Part model, mm, in its own coordinate system. A direction names the side the tool comes from. Give positions to 0.01 mm unless a question says otherwise; leave off trailing zeros. Write each loop counter-clockwise with the first axis right and the second up, starting at its lowest first coordinate (ties: lowest second). Pieces come first, ordered by that corner, then holes.
from build123d import *

# Parameters (mm, degrees)
ESQUISSE2_R                  = 20
BOSS_EXTRU_1_DEPTH           = 5
BOSS_EXTRU_2_DEPTH           = 5
R_P_TITION_CIRCULAIRE1_COUNT = 24
D_GAGEMENT_M22_D             = 5.1
BOSS_EXTRU_3_DEPTH           = 7.5
ENL_V_MAT_EXTRU_2_DEPTH      = 83.82071633
ENL_V_MAT_EXTRU_2_DEPTH_BACK = 83.82071633
ESQUISSE13_W                 = 57.206213055
ESQUISSE13_H                 = 37.798612504
ESQUISSE14_W                 = 4.5
ESQUISSE14_H                 = 4.5
BOSS_EXTRU_5_DEPTH           = 5
ESQUISSE17_W                 = 20
ESQUISSE17_H                 = 15
BOSS_EXTRU_7_DEPTH           = 2
CONG_1_R                     = 2
CONG_2_R                     = 2


with BuildPart() as part:
    # Esquisse2 → Boss.-Extru.1 (new body)
    with BuildSketch(Plane(origin=(0, 0, 0), x_dir=(1, 0, 0), z_dir=(0, 1, 0))):
        with Locations(Location((0, 0, 0), (0, 0, 270))):
            Circle(ESQUISSE2_R)
    extrude(amount=BOSS_EXTRU_1_DEPTH)

    # Esquisse3 → Boss.-Extru.2 (add)
    with BuildSketch(Plane(origin=(0, 5, 0), x_dir=(1, 0, 0), z_dir=(0, 1, 0))):
        Polygon((-1.625, 19.933875062), (-1.25, 21.933875062), (1.25, 21.933875062), (1.625, 19.933875062), align=None)
    boss_extru_2 = extrude(amount=-BOSS_EXTRU_2_DEPTH)

    # Répétition circulaire1: Boss.-Extru.2 ×24 about axis
    r_p_tition_circulaire1_axis = Axis((0, 0, 0), (0, 1, 0))
    for i in range(1, R_P_TITION_CIRCULAIRE1_COUNT):
        add(boss_extru_2.rotate(r_p_tition_circulaire1_axis, i * 360 / R_P_TITION_CIRCULAIRE1_COUNT))

    # Dégagement M22 (through all)
    with Locations(Plane(origin=(0, 5, 0), x_dir=(1, 0, 0), z_dir=(0, 1, 0))):
        with Locations((0, 0)):
            Hole(D_GAGEMENT_M22_D / 2)

    # Esquisse11 → Boss.-Extru.3 (add)
    with BuildSketch(Plane(origin=(0, 5, 0), x_dir=(1, 0, 0), z_dir=(0, 1, 0))):
        Polygon((-5.801101772, -14.332121903), (1.625908743, -15.37592016), (-0.461687771, -30.229941191), (3.284378163, -39.501779737), (-2.282545875, -79.112502486), (-6.738752185, -78.486223532), (-1.894992792, -44.021084607), (-7.888698287, -29.186142934), align=None)
    extrude(amount=-BOSS_EXTRU_3_DEPTH)

    # Esquisse13 → Enlèv. mat.-Extru.2 (cut, two sides: drawn at the far end of the back side and taken through both)
    with BuildSketch(Plane(origin=(3.713505258, 0, 0.521899129), x_dir=(0.13917310096006574, 0, -0.9902680687415703), z_dir=(0.9902680687415703, 0, 0.13917310096006574)).offset(-ENL_V_MAT_EXTRU_2_DEPTH_BACK)):
        with Locations((6.964953995, 7.661661133)):
            Rectangle(ESQUISSE13_W, ESQUISSE13_H)
    extrude(amount=ENL_V_MAT_EXTRU_2_DEPTH + ENL_V_MAT_EXTRU_2_DEPTH_BACK, mode=Mode.SUBTRACT)

    # Esquisse14 → Boss.-Extru.5 (add)
    with BuildSketch(Plane(origin=(-3.011448787, 0, 21.427571519), x_dir=(-0.9902680687415703, 0, -0.13917310096006574), z_dir=(0.13917310096006574, 0, -0.9902680687415703))):
        with Locations((0, 1.25)):
            Rectangle(ESQUISSE14_W, ESQUISSE14_H)
    extrude(amount=BOSS_EXTRU_5_DEPTH)

    # Esquisse17 → Boss.-Extru.7 (add)
    with BuildSketch(Plane(origin=(8.664845601, 0, 1.217764633), x_dir=(0.13917310096006535, 0, -0.9902680687415704), z_dir=(0.9902680687415704, 0, 0.13917310096006535))):
        with Locations((-78.660254038, 1.25)):
            Rectangle(ESQUISSE17_W, ESQUISSE17_H)
    extrude(amount=-BOSS_EXTRU_7_DEPTH)

    # Congé1
    cong_1_edges = [part.edges().sort_by_distance(p)[0] for p in [
        (-3.567216508, -2.5, 73.882815941),
        (-3.567216508, 5, 73.882815941),
        (-4.263082013, 1.25, 78.834156284),
    ]]
    fillet(cong_1_edges, radius=CONG_1_R)

    # Congé2
    # the kernel refuses this fillet: 2 mm, written as the material it takes off along each edge
    with BuildSketch(Plane(origin=(-6.738752185, 9.270248109, 78.486223532), x_dir=(0.13917310096006505, 0, -0.9902680687415704), z_dir=(0, -1, 0))) as cong_2_piece_1:
        with BuildLine():
            CenterArc((1.708099244, 2), CONG_2_R, 202.024312837, 67.975687163)
            Line((-0.145950378, 1.25), (-0.33135534, 1.175))
            ThreePointArc((-0.33135534, 1.175), (-0.2, 0.5), (-0.2, 0))
            Line((-0.2, 0), (0, -0.2))
            Line((0, -0.2), (1.708099244, -0.2))
            Line((1.708099244, -0.2), (1.708099244, 0))
        make_face()
    extrude(amount=16.040496218, mode=Mode.SUBTRACT)


solid = part.part
1) Saw through at C-C (y = 1.25). Write the cut outline in (x, z) (1 decimal).
Check result:
outline: (-7.9, 29.2) - (-6.7, 20.9) - (-5.2, 21.1) - (-4.5, 16.2) - (-0.1, 16.8) - (-0.8, 21.7) - (0.7, 21.9) - (-0.5, 30.2) - (3.3, 39.5) - (-3.7, 89) - (-5.7, 88.7) - (-4.5, 80.8) arc R2 cw to (-5.5, 78.8) arc R2 ccw to (-6.5, 76.8) - (-1.9, 44) - close
2) Drill centre lines: L1, parallel to Y at x = -2.5, z = 65; L2, parallel to X at y = -5.25, z = 72; L3, parallel to X at y = 2.5, z = 54. Where is each one in solid material? Low to high.
Check result:
L1: y = -2.5 to 5
L2: x = -3.3 to -1.28
L3: x = -3.3 to 1.25
3) Flat gauge pins, fed straight in: P1, Ø2, axis at x = -4, z = 31, coming from the -Y side; P2, Ø5, axis at y = 3.5, z = 74, coming from the -X side; P3, Ø1.5, axis at x = -3.5, z = 20, coming from the +Y side. Where does each tip first touch, or does it go through?
Check result:
P1: stops at y = -2.5
P2: stops at x = -6.46
P3: stops at y = 3.5
4) 3-axis set-ups, long thin cutter, end or side, ignore diameter. For faces 5 (the flat face through (-1.96, 6.85, 69.06)), 6 (the flat face through (-4.85, 1.3, 36.71)), 7 (the cylindrical face through (-4.283, 5.601, 74.877)), 8 (the flat face through (-1.96, -4.4, 69.06)), 9 (the flat face through (0.13, 1.3, 26.03)): which of +Z, -Z, +X, -X, +Y, -Y reach the whole face in a straight line?
Check result:
face 5: -Z, +X, +Y
face 6: -X, +Y, -Y
face 7: -Z, -X, +Y
face 8: -Z, +X, -Y
face 9: +X, +Y, -Y
5) Mould opens along Z. For faces 1 (the flat face through (-2, 5, 41)), 2 (the flat face through (-4.65, 1.15, 88.88)), 3 (the flat face through (-4.9, 1.36, 83.37)), 4 (the flat face through (-4.9, 1.2, 18.7)) say: +Z half, -Z half, draft (parallel to the pull), parting line (faces both ways), or undercut.
Check result:
face 1: draft
face 2: +Z half
face 3: undercut
face 4: -Z half
6) Saw through at A-A (y = 7.75). Write the cut outline in (x, z), and give its area (3 significant figures).
Check result:
outline: (-5.65, 88.74) - (-2.87, 68.93) - (-0.89, 69.21) - (-3.67, 89.02) - close
area: 40.0 mm2
7) Saw through at B-B (z = 81.5). Write the cut outline in (x, y).
Check result:
outline: (-4.64, -6.25) - (-2.62, -6.25) - (-2.62, 8.75) - (-4.64, 8.75) - close
